For this review, take the finished solid that the model builds, in its own axes (mm). Face numbers are marked on the shaded views. A direction names the side the tool comes from. Give positions to 0.01 mm unless a question says otherwise; leave off trailing zeros. Order: outer loops, then holes, each group sorted by start corner. A loop starts at its lowest first (then second) coordinate and runs counter-clockwise, first axis right, second up. Notation, with made-up numbers: (81, 45.5) - (129, 45.5) arc R12 cw to (129, 68.5) - close; hole circle Ø3 at (43.5, 60). An arc over 180 degrees is marked (long way). Use a Markdown table: item, result. Add a question column.
1) Machinability: for the marked faces 4 and 5, which of the approach directions +Z, -Z, +X, -X, +Y, -Y give a long, thin tool a straight path to every point of the face, cutting with its end or side? Answer none if there is none.
2) Wall thickness on L1, parallel to X at y = -23, z = 1.75; L2, parallel to Y at x = 21.5, z = 3.5; L3, parallel to X at y = 1, z = -1: over which ranges is each line inside the solid? List them lowest first.
3) We need section A-A on y = 0. Give the number of separate pieces and of enclosed holes in the cut face, then the cut area to 3 significant figures.
4) Clearance check with flat-ended pins moving along their axes: P1, Ø6, axis at x = -5.5, z = 1.5, coming from the +Y side; P2, Ø5, axis at y = 6, z = 0, coming from the -X side; P3, Ø8, axis at x = 21, z = -3, coming from the -Y side. State where each tip first meets the part, or that it passes through.
5) Mouldability with a two-part tool opening along Y and no side actions: class the marked faces 1, 2 and 3 as released by +Y, released by -Y, zero draft, split by the parting line, or undercut.
6) We need section B-B on x = 12. Write out the cut boundary in (y, z).
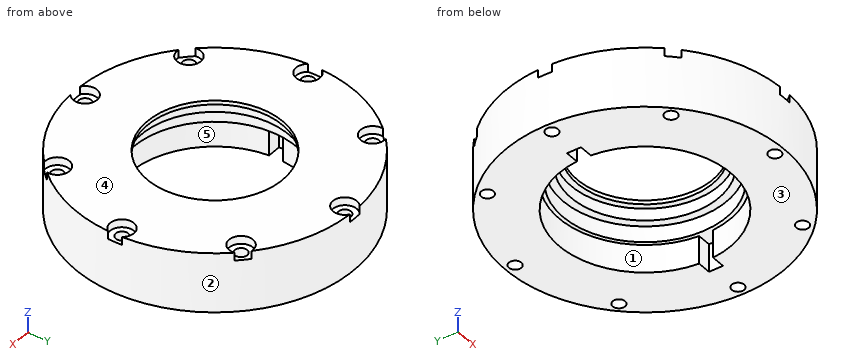
```python
from build123d import *

# Parameters (mm, degrees)
SKETCH_1_R          = 35
SKETCH_1_R_2        = 18.5
EXTRUDE_1_DEPTH     = 3
SKETCH_5_R          = 35
SKETCH_5_R_2        = 17
EXTRUDE_3_DEPTH     = 1
EXTRUDE_START       = 4
SKETCH_7_R          = 35
SKETCH_7_R_2        = 21.45
EXTRUDE_4_DEPTH     = 4
EXTRUDE_START_2     = 7
SKETCH_9_R          = 35
EXTRUDE_6_DEPTH     = 7
SKETCH_12_R         = 1.55
CUT_EXTRUDE_1_DEPTH = 52.720402164
SKETCH_13_R         = 3
CUT_EXTRUDE_2_DEPTH = 2
SKETCH_15_R         = 1.55
CUT_EXTRUDE_3_DEPTH = 52.720402164
SKETCH_16_R         = 3
CUT_EXTRUDE_4_DEPTH = 2
SKETCH_17_R         = 21.45
SKETCH_17_R_2       = 20.5
EXTRUDE_7_DEPTH     = 4


with BuildPart() as part:
    # 草图1 → 凸台-拉伸1 (new body)
    with BuildSketch(Plane.XY):
        Circle(SKETCH_1_R)
        Circle(SKETCH_1_R_2, mode=Mode.SUBTRACT)
    extrude(amount=EXTRUDE_1_DEPTH)

    # 草图5 → 凸台-拉伸3 (add)
    with BuildSketch(Plane.XY.offset(3)):
        Circle(SKETCH_5_R)
        Circle(SKETCH_5_R_2, mode=Mode.SUBTRACT)
    extrude(amount=EXTRUDE_3_DEPTH)

    # 草图7 → 凸台-拉伸4 (add)
    with BuildSketch(Plane(origin=(0, 0, 0), x_dir=(-1, 0, 0), z_dir=(0, 0, -1)).offset(EXTRUDE_START)):
        Circle(SKETCH_7_R)
        Circle(SKETCH_7_R_2, mode=Mode.SUBTRACT)
    extrude(amount=-EXTRUDE_4_DEPTH)

    # 草图9 → 凸台-拉伸6 (add)
    with BuildSketch(Plane(origin=(0, 0, -4), x_dir=(-1, 0, 0), z_dir=(0, 0, -1)).offset(EXTRUDE_START_2)):
        Circle(SKETCH_9_R)
        with BuildLine():
            Line((24.8, 1.75), (24.8, 0))
            Line((24.8, 0), (24.8, -1.75))
            Line((24.8, -1.75), (21.382497565, -1.75))
            ThreePointArc((21.382497565, -1.75), (0, -21.453990354), (-21.382497565, -1.75))
            Line((-21.382497565, -1.75), (-24.8, -1.75))
            Line((-24.8, -1.75), (-24.8, 1.75))
            Line((-24.8, 1.75), (-21.382497565, 1.75))
            ThreePointArc((-21.382497565, 1.75), (0, 21.453990354), (21.382497565, 1.75))
            Line((21.382497565, 1.75), (24.8, 1.75))
        make_face(mode=Mode.SUBTRACT)
    extrude(amount=-EXTRUDE_6_DEPTH)

    # 草图12 → 切除-拉伸1 (cut, through all)
    with BuildSketch(Plane.XY.offset(4)):
        with Locations((0, 32.5)):
            Circle(SKETCH_12_R)
        with Locations((-32.5, 0)):
            Circle(SKETCH_12_R)
        with Locations((0, -32.5)):
            Circle(SKETCH_12_R)
        with Locations((32.5, 0)):
            Circle(SKETCH_12_R)
    extrude(amount=-CUT_EXTRUDE_1_DEPTH, mode=Mode.SUBTRACT)

    # 草图13 → 切除-拉伸2 (cut)
    with BuildSketch(Plane.XY.offset(4)):
        with Locations((0, 32.5)):
            Circle(SKETCH_13_R)
        with Locations((32.5, 0)):
            Circle(SKETCH_13_R)
        with Locations((0, -32.5)):
            Circle(SKETCH_13_R)
        with Locations((-32.5, 0)):
            Circle(SKETCH_13_R)
    extrude(amount=-CUT_EXTRUDE_2_DEPTH, mode=Mode.SUBTRACT)

    # 草图15 → 切除-拉伸3 (cut, through all)
    with BuildSketch(Plane.XY.offset(4)):
        with Locations((22.980970389, 22.980970389)):
            Circle(SKETCH_15_R)
        with Locations((22.980970389, -22.980970389)):
            Circle(SKETCH_15_R)
        with Locations((-22.980970389, -22.980970389)):
            Circle(SKETCH_15_R)
        with Locations((-22.980970389, 22.980970389)):
            Circle(SKETCH_15_R)
    extrude(amount=-CUT_EXTRUDE_3_DEPTH, mode=Mode.SUBTRACT)

    # 草图16 → 切除-拉伸4 (cut)
    with BuildSketch(Plane.XY.offset(4)):
        with Locations((22.980970389, 22.980970389)):
            Circle(SKETCH_16_R)
        with Locations((22.980970389, -22.980970389)):
            Circle(SKETCH_16_R)
        with Locations((-22.980970389, -22.980970389)):
            Circle(SKETCH_16_R)
        with Locations((-22.980970389, 22.980970389)):
            Circle(SKETCH_16_R)
    extrude(amount=-CUT_EXTRUDE_4_DEPTH, mode=Mode.SUBTRACT)

    # 草图17 → 凸台-拉伸7 (add)
    with BuildSketch(Plane(origin=(0, 0, 0), x_dir=(-1, 0, 0), z_dir=(0, 0, -1)).offset(EXTRUDE_START)):
        Circle(SKETCH_17_R)
        Circle(SKETCH_17_R_2, mode=Mode.SUBTRACT)
    extrude(amount=-EXTRUDE_7_DEPTH)


solid = part.part
```
Checked values:
| question | item | result |
|---|---|---|
| 1 | face 4 | +Z, +X, -X, +Y, -Y |
| 1 | face 5 | -Z |
| 2 | L1 | -26.38 to -24.53, -21.43 to 21.43, 24.53 to 26.38 |
| 2 | L2 | -27.62 to -25.59, -20.37 to 20.37, 25.59 to 27.62 |
| 2 | L3 | -34.99 to -33.68, -31.32 to -20.48, 20.48 to 31.32, 33.68 to 34.99 |
| 3 | separate pieces | 4 |
| 3 | enclosed holes | 0 |
| 3 | area | 291 mm² |
| 4 | P1 | y = 34.91 |
| 4 | P2 | x = -34.82 |
| 4 | P3 | y = -30.59 |
| 5 | face 1 | undercut |
| 5 | face 2 | split by the parting line |
| 5 | face 3 | zero draft |
| 6 | outline | (-32.88, -11) - (-17.78, -11) - (-17.78, -4) - (-16.62, -4) - (-16.62, 0) - (-14.08, 0) - (-14.08, 3) - (-12.04, 3) - (-12.04, 4) - (-32.88, 4) - close; (12.04, 3) - (14.08, 3) - (14.08, 0) - (16.62, 0) - (16.62, -4) - (17.78, -4) - (17.78, -11) - (32.88, -11) - (32.88, 4) - (12.04, 4) - close |
